Autodesk Inventor part; units mm, degrees
ref_plane "YZ Plane" through (0, 0, 0) normal (1, 0, 0) x (0, 1, 0)
ref_plane "XZ Plane" through (0, 0, 0) normal (0, 1, 0) x (-1, 0, 0)
ref_plane "XY Plane" through (0, 0, 0) normal (0, 0, 1) x (1, 0, 0)
sketch "Szkic1" plane through (0, 0, 0) normal (0, 1, 0) x (-1, 0, 0)
  line L0 (0, 0) -> (42.5, 0)
  line L1 (42.5, 0) -> (42.5, 20.5)
  line L2 (42.5, 20.5) -> (0, 20.5)
  line L3 (0, 20.5) -> (0, 0)
  line L4 (42.5, 20.5) -> (44, 20.5) construction
  line L5 (44, 20.5) -> (44, 22) construction
  line L6 (44, 22) -> (-1.5, 22)
  line L7 (-1.5, 22) -> (-1.5, -1.5)
  line L8 (-1.5, -1.5) -> (44, -1.5)
  line L9 (44, -1.5) -> (44, 22)
  line L10 (42.5, 20.5) -> (37.5, 20.5) construction
  line L11 (0, 20.5) -> (5, 20.5) construction
  line L12 (37.5, 20.5) -> (33.5, 20.5)
  line L13 (33.5, 20.5) -> (33.5, 16.5)
  line L14 (33.5, 16.5) -> (37.5, 16.5)
  line L15 (37.5, 16.5) -> (37.5, 20.5)
  line L16 (5, 20.5) -> (9, 20.5)
  line L17 (9, 20.5) -> (9, 16.5)
  line L18 (9, 16.5) -> (5, 16.5)
  line L19 (5, 16.5) -> (5, 20.5)
  line L20 (37.5, 0) -> (33.5, 0)
  line L21 (33.5, 0) -> (33.5, 4)
  line L22 (33.5, 4) -> (37.5, 4)
  line L23 (37.5, 4) -> (37.5, 0)
  line L24 (5, 0) -> (9, 0)
  line L25 (9, 0) -> (9, 4)
  line L26 (9, 4) -> (5, 4)
  line L27 (5, 4) -> (5, 0)
  dimension "d0" = 42.5
  dimension "d1" = 20.5
  dimension "d2" = 1.5
  dimension "d3" = 1.5
  dimension "d4" = 45.5
  dimension "d5" = 23.5
  dimension "d6" = 5
  dimension "d7" = 5
  dimension "d8" = 4
  dimension "d9" = 4
  dimension "d10" = 4
  dimension "d11" = 4
  dimension "d12" = 4
  dimension "d13" = 4
  dimension "d14" = 4
  dimension "d15" = 4
extrude "Wyciągnięcie proste1" add sketch "Szkic1" along normal blind 1.5 contours L3 L2 L19 L18 L17 L13 L14 L15 L1 L0 L23 L22 L21 L25 L26 L27
sketch "Szkic2" plane through (0, 0, 0) normal (0, -1, 0) x (1, 0, 0)
  line L0 (-5, 4) -> (-5, 0)
  line L1 (-5, 0) -> (-9, 0)
  line L2 (-9, 0) -> (-9, 4)
  line L3 (-9, 4) -> (-5, 4)
  line L4 (-5, 4) -> (-5, 0)
  line L5 (-33.5, 0) -> (-33.5, 4)
  line L6 (-33.5, 0) -> (-37.5, 0)
  line L7 (-37.5, 0) -> (-37.5, 4)
  line L8 (-37.5, 4) -> (-33.5, 4)
  line L9 (-33.5, 4) -> (-33.5, 0)
  line L10 (-37.5, 20.5) -> (-37.5, 16.5)
  line L11 (-33.5, 16.5) -> (-37.5, 16.5)
  line L12 (-37.5, 16.5) -> (-37.5, 20.5)
  line L13 (-37.5, 20.5) -> (-33.5, 20.5)
  line L14 (-33.5, 20.5) -> (-33.5, 16.5)
  line L15 (-5, 16.5) -> (-5, 20.5)
  line L16 (-33.5, 20.5) -> (-9, 20.5)
  line L17 (-5, 16.5) -> (-9, 16.5)
  line L18 (-9, 16.5) -> (-9, 20.5)
  line L19 (-9, 20.5) -> (-5, 20.5)
  line L20 (-5, 20.5) -> (-5, 16.5)
  point P0 (0, 0)
extrude "Wyciągnięcie proste2" add sketch "Szkic2" against normal blind 3
sketch "Szkic3" plane through (0, 0, 0) normal (0, -1, 0) x (1, 0, 0)
  line L0 (-42.5, 0) -> (-42.5, -1.5) construction
  line L1 (-42.5, -1.5) -> (-44, -1.5) construction
  line L2 (-44, -1.5) -> (1.5, -1.5)
  line L3 (1.5, -1.5) -> (1.5, 22)
  line L4 (1.5, 22) -> (-44, 22)
  line L5 (-44, 22) -> (-44, -1.5)
  line L6 (-42.5, 0) -> (0, 0)
  line L7 (0, 0) -> (0, 20.5)
  line L8 (0, 20.5) -> (-42.5, 20.5)
  line L9 (-42.5, 20.5) -> (-42.5, 0)
  dimension "d20" = 1.5
  dimension "d21" = 1.5
  dimension "d22" = 45.5
  dimension "d23" = 23.5
extrude "Wyciągnięcie proste3" add sketch "Szkic3" against normal blind 17
sketch "Szkic4" plane through (-44, 0, -1.5) normal (-1, 0, 0) x (0, 0, 1)
  line L0 (23.5, 0) -> (0, 0) construction
  line L1 (0, 0) -> (11.75, 0) construction
  line L2 (11.75, 0) -> (11.75, 3) construction
  line L3 (11.75, 3) -> (15.25, 3) construction
  line L4 (15.25, 3) -> (15.25, 7) construction
  line L5 (15.25, 7) -> (8.25, 7)
  line L6 (8.25, 7) -> (8.25, 3)
  line L7 (8.25, 3) -> (15.25, 3)
  line L8 (15.25, 3) -> (15.25, 7)
  point P0 (1.5, 0)
  dimension "d26" = 3
  dimension "d27" = 3.5
  dimension "d28" = 4
  dimension "d29" = 7
  dimension "d30" = 4
extrude "Wyciągnięcie proste4" cut sketch "Szkic4" against normal blind 50
properties part number "dol"
Read the model definition and answer for the solid it produces. Units are mm, in the model's axes. A direction names the side the tool comes from. Give positions to 0.01 mm unless a question says otherwise; leave off trailing zeros. Write each loop counter-clockwise with the first axis right and the second up, starting at its lowest first coordinate (ties: lowest second). Pieces come first, ordered by that corner, then holes. Notation, with made-up numbers: (26.25, 3) -> (76.25, 3) arc R21 cw to (76.25, 8) -> close; hole circle Ø2 at (50, 55.5). An arc over 180 degrees is marked (long way). Answer as a JSON object with one key per item and string values. Group by question number.
1) Find section B-B (z = 12.25). Write down the section's boundary in (x, y).
2) The mould has two halves that part along Y. Classify faces 4 (the flat face through (-36, 3, 2)), 5 (the flat face through (-43, 7, 10)), 6 (the flat face through (-37.5, 2, 2)): +Y half, -Y half, draft (parallel to the pull), parting line (faces both ways), or undercut.
3) Find section C-C (y = 14.25). Write down the section's boundary in (x, z).
4) Find section D-D (x = -39). Write down the section's boundary in (y, z), and give its area (4 significant figures).
5) Consider L1, parallel to Z at x = -2.5, y = 11.5; L2, parallel to X at y = 14, z = 6; L3, parallel to Y at x = -31, z = 18.5. Determine where each line is inside the solid, lowest interval first. Write a range as from..to.
6) Find section A-A (y = 6.5). Write down the section's boundary in (x, z), and give its area (3 significant figures).
7) A tool of negligible diameter and unlimited length cuts with its end or side. For faces 1 (the flat face through (-5, 2, 18)), 2 (the flat face through (-43, 5, 6.75)), 3 (the flat face through (1.5, 8, 10)), from which of +Z, -Z, +X, -X, +Y, -Y can it reach the whole face along a straight path? Write none if from no direction.
8) Each of these flat-tipped pins is pushed along its axis until it touches: P1, Ø4.5, axis at x = -35, z = 18, coming from the +Y side; P2, Ø6, axis at x = -20.5, z = 14.5, coming from the +Y side. Where does it stop, or does it pass through?
Values follow:
{
 "1": {"outline": "(-44, 0) -> (1.5, 0) -> (1.5, 3) -> (0, 3) -> (0, 1.5) -> (-42.5, 1.5) -> (-42.5, 3) -> (-44, 3) -> close; (-44, 7) -> (-42.5, 7) -> (-42.5, 17) -> (-44, 17) -> close; (0, 7) -> (1.5, 7) -> (1.5, 17) -> (0, 17) -> close"},
 "2": {"face 4": "+Y half", "face 5": "undercut", "face 6": "draft"},
 "3": {"outline": "(-44, -1.5) -> (1.5, -1.5) -> (1.5, 22) -> (-44, 22) -> close; hole (-42.5, 0) -> (0, 0) -> (0, 20.5) -> (-42.5, 20.5) -> close"},
 "4": {"outline": "(0, -1.5) -> (17, -1.5) -> (17, 0) -> (1.5, 0) -> (1.5, 20.5) -> (17, 20.5) -> (17, 22) -> (0, 22) -> close", "area": "81.75 mm2"},
 "5": {"L1": "z = -1.5..0, 20.5..22", "L2": "x = -44..-42.5, 0..1.5", "L3": "y = 0..1.5"},
 "6": {"outline": "(-44, -1.5) -> (1.5, -1.5) -> (1.5, 6.75) -> (0, 6.75) -> (0, 0) -> (-42.5, 0) -> (-42.5, 6.75) -> (-44, 6.75) -> close; (-44, 13.75) -> (-42.5, 13.75) -> (-42.5, 20.5) -> (0, 20.5) -> (0, 13.75) -> (1.5, 13.75) -> (1.5, 22) -> (-44, 22) -> close", "area": "177 mm2"},
 "7": {"face 1": "+Y", "face 2": "+X, -X", "face 3": "+Z, -Z, +X, +Y, -Y"},
 "8": {"P1": "stops at y = 3", "P2": "stops at y = 1.5"}
}
